from build123d import *
from OCP.BRepAlgoAPI import BRepAlgoAPI_Cut
from OCP.TopTools import TopTools_ListOfShape

# Parameters (mm, degrees)
EXTRUDE_START       = -40
EXTRUDE_1_DEPTH     = 80
SKETCH_2_R          = 4
CUT_EXTRUDE_1_DEPTH = 99.895232583
SKETCH_3_R          = 3
CUT_EXTRUDE_2_DEPTH = 99.895232848
SWEEP_6_PROFILE_R   = 2.5


with BuildPart() as part:
    # 凸台-拉伸1: read off the stored shape, not the designer's step
    # 凸台-拉伸1 outline → 凸台-拉伸1 (new body)
    with BuildSketch(Plane(origin=(0, 0, 0), x_dir=(0, 0, -1), z_dir=(1, 0, 0)).offset(EXTRUDE_START)):
        with BuildLine():
            Line((-1.999999781, -5.28e-07), (8.38e-07, -5.28e-07))
            Line((8.38e-07, -5.28e-07), (8.38e-07, 54.999999472))
            ThreePointArc((8.38e-07, 54.999999472), (-1.464465344, 58.535533909), (-4.999999781, 60.000000091))
            Line((-4.999999781, 60.000000091), (-49.999999781, 60.000000091))
            ThreePointArc((-49.999999781, 60.000000091), (-51.913417169, 59.619397955), (-53.535534, 58.535534))
            Line((-53.535534, 58.535534), (-67.67767, 44.393398))
            Line((-67.67767, 44.393398), (-66.262742, 42.978678))
            Line((-66.262742, 42.978678), (-52.12132, 57.12132))
            ThreePointArc((-52.12132, 57.12132), (-51.148050068, 57.771638319), (-49.999999781, 57.999999472))
            Line((-49.999999781, 57.999999472), (-4.999999781, 57.999999472))
            ThreePointArc((-4.999999781, 57.999999472), (-2.878679344, 57.121319909), (-1.999999781, 54.999999472))
            Line((-1.999999781, 54.999999472), (-1.999999781, -5.28e-07))
        make_face()
    extrude(amount=EXTRUDE_1_DEPTH)


with BuildPart() as cut_extrude_1_tool:
    # 草图2 → 切除-拉伸1 (new, through all)
    with BuildSketch(Plane.XY):
        with Locations(Location((0, 25, 0), (0, 0, 180))):
            Circle(SKETCH_2_R)
    extrude(amount=CUT_EXTRUDE_1_DEPTH)


with BuildPart() as part_1:
    add(part.part)

    # 切除-拉伸1: cut by cut_extrude_1_tool, with a tolerance
    cut_extrude_1_stock = TopTools_ListOfShape()
    cut_extrude_1_stock.Append(part_1.part.wrapped)
    cut_extrude_1_tools = TopTools_ListOfShape()
    cut_extrude_1_tools.Append(cut_extrude_1_tool.part.wrapped)
    cut_extrude_1_cut = BRepAlgoAPI_Cut()
    cut_extrude_1_cut.SetArguments(cut_extrude_1_stock)
    cut_extrude_1_cut.SetTools(cut_extrude_1_tools)
    cut_extrude_1_cut.SetFuzzyValue(0.00001)
    cut_extrude_1_cut.Build()
    add(Compound.cast(cut_extrude_1_cut.Shape()).solids(), mode=Mode.REPLACE)

    # 草图3 → 切除-拉伸2 (cut, through all)
    with BuildSketch(Plane(origin=(0, 60, 0), x_dir=(1, 0, 0), z_dir=(0, 1, 0))):
        with Locations(Location((-25, -24.031, 0), (0, 0, 270))):
            Circle(SKETCH_3_R)
        with Locations(Location((25, -24.031, 0), (0, 0, 270))):
            Circle(SKETCH_3_R)
    extrude(amount=-CUT_EXTRUDE_2_DEPTH, mode=Mode.SUBTRACT)

    # 切除-扫描6: sweep along a curve in space
    with BuildLine() as sweep_6_path:
        Line((0, 53.11, 62.755), (0, 46.038932, 55.683932))
    # 切除-扫描6 profile (on start of the path) → 切除-扫描6 (sweep, cut)
    with BuildSketch(Plane(origin=(0, 53.11, 62.755), x_dir=(0, -0.7071067811865479, 0.7071067811865471), z_dir=(0, -0.7071067811865471, -0.7071067811865479))):
        Circle(SWEEP_6_PROFILE_R)
    sweep(path=sweep_6_path.line, mode=Mode.SUBTRACT)


solid = part_1.part
Design review of the part built by this model. Coordinates are the model's own, in mm. A direction names the side the tool comes from. Round coordinates to 2 decimals unless told otherwise and drop trailing zeros. Write each loop counter-clockwise with the first axis right and the second up, starting at its lowest first coordinate (ties: lowest second). Pieces come first, ordered by that corner, then holes. Notation, with made-up numbers: (74.25, 2.5) - (102.25, 2.5) arc R29 cw to (102.25, 41.5) - close; hole circle Ø11 at (-34.5, -29.75). An arc over 180 degrees is marked (long way). Return JSON: item names as keys, results as strings. Group by question number.
Item 1: We need section B-B on y = 25. Write out the cut boundary in (x, z).
Item 2: For probe 1 along Z at (x, y) = (19.5, 7); probe 2 along X at (y, z) = (25, 1); probe 3 along Y at (x, z) = (34, 15), list the stretches that pass through material, from the lowest coordinate up. Write a range as [from, to].
Item 3: Insertion check: P1, Ø22.5, axis at x = -15, z = 31.5, coming from the -Y side; P2, Ø5.5, axis at x = -25, z = 24.031, coming from the +Y side; P3, Ø5, axis at x = 14, y = 28.5, coming from the +Z side. Each pin has a flat end and moves straight along its axis. Give the tip position at first contact, or say it passes through.
Item 4: We need section A-A on x = 25. Write out the cut boundary in (y, z), and give its area (3 significant figures).
Item 5: The part is to be moulded in two halves that separate along X. For faces 3 (the face through (40, 59, 19)), 4 (the face through (-0.56, 57.14, 2.9)), 5 (the face through (-24.868, 59.014, 21.034)), say which applies: pulls with the +X half, pulls with the -X half, needs draft (parallel to the pull), parting line crosses it, or undercut.
Item 6: Machinability: for faces 1 (the face through (-1, 60, 27)), 2 (the face through (-1, 58, 28)), which of the approach directions +Z, -Z, +X, -X, +Y, -Y give a long, thin tool a straight path to every point of the face, cutting with its end or side? Answer none if there is none.
Item 7: We need section D-D on x = -10. Write out the cut boundary in (y, z).
Item 8: We need section C-C on x = 0. Write out the cut boundary in (y, z), and give its area (3 significant figures).
Model answer:
{
 "1": {"outline": "(-40, 0) - (-4, 0) - (-4, 2) - (-40, 2) - close; (4, 0) - (40, 0) - (40, 2) - (4, 2) - close"},
 "2": {"probe 1": "z = [0, 2]", "probe 2": "x = [-40, -4], [4, 40]", "probe 3": "y = [58, 60]"},
 "3": {"P1": "stops at y = 58", "P2": "passes through", "P3": "stops at z = 2"},
 "4": {"outline": "(0, 0) - (55, 0) arc R5 ccw to (60, 5) - (60, 21.03) - (58, 21.03) - (58, 5) arc R3 cw to (55, 2) - (0, 2) - close; (42.98, 66.26) - (57.12, 52.12) arc R3 cw to (58, 50) - (58, 27.03) - (60, 27.03) - (60, 50) arc R5 ccw to (58.54, 53.54) - (44.39, 67.68) - close", "area": "247 mm²"},
 "5": {"face 3": "pulls with the +X half", "face 4": "needs draft", "face 5": "undercut"},
 "6": {"face 1": "+Z, -Z, +X, -X, +Y", "face 2": "+X, -X, -Y"},
 "7": {"outline": "(0, 0) - (55, 0) arc R5 ccw to (60, 5) - (60, 50) arc R5 ccw to (58.54, 53.54) - (44.39, 67.68) - (42.98, 66.26) - (57.12, 52.12) arc R3 cw to (58, 50) - (58, 5) arc R3 cw to (55, 2) - (0, 2) - close"},
 "8": {"outline": "(0, 0) - (21, 0) - (21, 2) - (0, 2) - close; (29, 0) - (55, 0) arc R5 ccw to (60, 5) - (60, 50) arc R5 ccw to (58.54, 53.54) - (52.98, 59.09) - (51.57, 57.68) - (57.12, 52.12) arc R3 cw to (58, 50) - (58, 5) arc R3 cw to (55, 2) - (29, 2) - close; (42.98, 66.26) - (48.03, 61.21) - (49.45, 62.63) - (44.39, 67.68) - close", "area": "233 mm²"}
}
